Check sheet for the modelled part. Datum: model origin and axes. Units: mm. A direction names the side the tool comes from. Round coordinates to 2 decimals unless told otherwise and drop trailing zeros. Write each loop counter-clockwise with the first axis right and the second up, starting at its lowest first coordinate (ties: lowest second). Pieces come first, ordered by that corner, then holes. Notation, with made-up numbers: (70.5, -3) -> (110.5, -3) arc R21 ccw to (110.5, 20) -> close; hole circle Ø11 at (23, -8). An arc over 180 degrees is marked (long way). One line per item, written item: value.
from build123d import *

# Parameters (mm, degrees)
SKETCH_1_R             = 0.5
EXTRUDE_1_DEPTH        = 10
HOLE_WIZARD_M3_1_D     = 2.5
HOLE_WIZARD_M3_1_DEPTH = 18.5
HOLE_WIZARD_M3_1_TIP   = 0.751075774
SKETCH_4_R             = 0.5
EXTRUDE_2_DEPTH        = 10
HOLE_WIZARD_M3_2_D     = 2.5
HOLE_WIZARD_M3_2_DEPTH = 18.5
HOLE_WIZARD_M3_2_TIP   = 0.751075774
SKETCH_6_W             = 18
SKETCH_6_H             = 9
CUT_EXTRUDE_1_DEPTH    = 0.5
EXTRUDE_3_DEPTH        = 0.5
EXTRUDE_4_DEPTH        = 2
FILLET_4_R             = 1
SKETCH_10_R            = 1
EXTRUDE_5_DEPTH        = 1
SKETCH_11_W            = 12
SKETCH_11_H            = 7
EXTRUDE_6_DEPTH        = 0.1
SKETCH_12_R            = 1
EXTRUDE_7_DEPTH        = 1
SKETCH_13_R            = 1.75
EXTRUDE_8_DEPTH        = 7
DRAFT_1_ANGLE          = 5


with BuildPart() as part:
    # 草图1 → 凸台-拉伸1 (new body)
    with BuildSketch(Plane(origin=(0, 0, 0), x_dir=(1, 0, 0), z_dir=(0, 1, 0))):
        with BuildLine():
            Line((-12.5, 10), (-17.5, 5))
            Line((-17.5, 5), (-17.5, -7.5))
            ThreePointArc((-17.5, -7.5), (-16.767766953, -9.267766953), (-15, -10))
            Line((-15, -10), (15, -10))
            ThreePointArc((15, -10), (16.767766953, -9.267766953), (17.5, -7.5))
            Line((17.5, -7.5), (17.5, 9.5))
            ThreePointArc((17.5, 9.5), (17.353553391, 9.853553391), (17, 10))
            Line((17, 10), (-12.5, 10))
        make_face()
        with Locations((-15, -7.5)):
            Circle(SKETCH_1_R, mode=Mode.SUBTRACT)
    extrude(amount=EXTRUDE_1_DEPTH)

    # M3 螺纹孔1
    with Locations(Plane(origin=(10, 10, 7.5), x_dir=(0, 0, 1), z_dir=(0, 1, 0))):
        with Locations((0, 0)):
            Hole(HOLE_WIZARD_M3_1_D / 2, depth=HOLE_WIZARD_M3_1_DEPTH)
            with Locations((0, 0, -(HOLE_WIZARD_M3_1_DEPTH + HOLE_WIZARD_M3_1_TIP / 2))):  # 118° drill point
                Cone(0, HOLE_WIZARD_M3_1_D / 2, HOLE_WIZARD_M3_1_TIP, mode=Mode.SUBTRACT)

    # 草图4 → 凸台-拉伸2 (add)
    with BuildSketch(Plane.XZ):
        with Locations((-15, 7.5)):
            Circle(SKETCH_4_R)
    extrude(amount=-EXTRUDE_2_DEPTH)

    # M3 螺纹孔2
    with Locations(Plane(origin=(-15, 10, 7.5), x_dir=(0, 0, 1), z_dir=(0, 1, 0))):
        with Locations((0, 0)):
            Hole(HOLE_WIZARD_M3_2_D / 2, depth=HOLE_WIZARD_M3_2_DEPTH)
            with Locations((0, 0, -(HOLE_WIZARD_M3_2_DEPTH + HOLE_WIZARD_M3_2_TIP / 2))):  # 118° drill point
                Cone(0, HOLE_WIZARD_M3_2_D / 2, HOLE_WIZARD_M3_2_TIP, mode=Mode.SUBTRACT)

    # 草图6 → 切除-拉伸1 (cut)
    with BuildSketch(Plane.XY.offset(10)):
        with Locations((-2, 5)):
            Rectangle(SKETCH_6_W, SKETCH_6_H)
    extrude(amount=-CUT_EXTRUDE_1_DEPTH, mode=Mode.SUBTRACT)

    # 草图8 → 凸台-拉伸3 (add)
    with BuildSketch(Plane(origin=(17.5, 0, 0), x_dir=(0, 0, -1), z_dir=(1, 0, 0))):
        with BuildLine():
            Line((8, 8.5), (-6, 8.5))
            ThreePointArc((-6, 8.5), (-6.353553391, 8.353553391), (-6.5, 8))
            Line((-6.5, 8), (-6.5, 2))
            ThreePointArc((-6.5, 2), (-6.353553391, 1.646446609), (-6, 1.5))
            Line((-6, 1.5), (8, 1.5))
            ThreePointArc((8, 1.5), (8.353553391, 1.646446609), (8.5, 2))
            Line((8.5, 2), (8.5, 8))
            ThreePointArc((8.5, 8), (8.353553391, 8.353553391), (8, 8.5))
        make_face()
    extrude(amount=EXTRUDE_3_DEPTH)

    # 草图9 → 凸台-拉伸4 (add)
    with BuildSketch(Plane(origin=(18, 0, 0), x_dir=(0, 0, -1), z_dir=(1, 0, 0))):
        with BuildLine():
            Line((-2, 6.5), (-2, 3.5))
            ThreePointArc((-2, 3.5), (-3.5, 2), (-5, 3.5))
            Line((-5, 3.5), (-5, 6.5))
            ThreePointArc((-5, 6.5), (-3.5, 8), (-2, 6.5))
        make_face()
    extrude(amount=EXTRUDE_4_DEPTH)

    # 圆角4
    fillet_4_edges = [part.edges().sort_by_distance(p)[0] for p in [
        (20, 8, 3.5),
        (20, 5, 5),
        (20, 2, 3.5),
        (20, 5, 2),
    ]]
    fillet(fillet_4_edges, radius=FILLET_4_R)

    # 草图10 → 凸台-拉伸5 (add)
    with BuildSketch(Plane(origin=(18, 0, 0), x_dir=(0, 0, -1), z_dir=(1, 0, 0))):
        with Locations((3.5, 5)):
            Circle(SKETCH_10_R)
    extrude(amount=EXTRUDE_5_DEPTH)

    # 草图11 → 凸台-拉伸6 (add)
    with BuildSketch(Plane(origin=(0, 0, -10), x_dir=(-1, 0, 0), z_dir=(0, 0, -1))):
        with Locations((-2.25, 5)):
            Rectangle(SKETCH_11_W, SKETCH_11_H)
    extrude(amount=EXTRUDE_6_DEPTH)

    # 草图12 → 凸台-拉伸7 (add)
    with BuildSketch(Plane(origin=(0, 0, -10), x_dir=(-1, 0, 0), z_dir=(0, 0, -1))):
        with Locations((-11.25, 5)):
            Circle(SKETCH_12_R)
        with Locations((6.75, 5)):
            Circle(SKETCH_12_R)
    extrude(amount=EXTRUDE_7_DEPTH)

    # 草图13 → 凸台-拉伸8 (add)
    with BuildSketch(Plane(origin=(-11.25, 0, -11.25), x_dir=(-0.707106781, 0, 0.707106781), z_dir=(-0.707106781, 0, -0.707106781))):
        with Locations((5.303300859, 5)):
            Circle(SKETCH_13_R)
    extrude(amount=EXTRUDE_8_DEPTH)

    # 拔模1
    draft_1_faces = [part.faces().sort_by_distance(p)[0] for p in [
        (-16.237436867, 5, -11.212310601),
    ]]
    draft(draft_1_faces, Plane(origin=(-19.949747468, 5, -12.449747468), x_dir=(-0.707106781, 0, 0.707106781), z_dir=(-0.707106781, 0, -0.707106781)), DRAFT_1_ANGLE)


solid = part.part
Item 1: Sectioned sample at C-C (x = -6.75). Enter the section's corners in (y, z), then the cut area to 4 significant figures.
Result set:
outline: (0, -10) -> (4, -10) -> (4, -11) -> (6, -11) -> (6, -10) -> (10, -10) -> (10, 10) -> (9.5, 10) -> (9.5, 9.5) -> (0.5, 9.5) -> (0.5, 10) -> (0, 10) -> close
area: 197.5 mm^2
Item 2: Depth check by flat-ended pin: pin 1 (1 mm diameter, centred on y = 4.5, z = -4, fed in from +X); pin 2 (2 mm diameter, centred on y = 5, z = 3, fed in from -X); pin 3 (4.5 mm diameter, centred on x = -1.5, y = 4.5, fed in from +Z). Enter the tip coordinate at first touch or a pass-through.
Result set:
pin 1: x = 19
pin 2: x = -17.5
pin 3: z = 9.5
Item 3: Release check for a two-part mould opening along X. For faces 4 (the flat face through (-17.5, 5, 1)), 5 (the flat face through (0, 0, 0)), 6 (the conical face through (-16.366, 6.393, -11.014)) record: pulls with the +X half, pulls with the -X half, needs draft (parallel to the pull), parting line crosses it, or undercut.
Result set:
face 4: pulls with the -X half
face 5: needs draft
face 6: undercut
Item 4: Tool access check on faces 1 (the cylindrical face through (18.5, 8, 3.5)), 2 (the cylindrical face through (18.493, 5.676, -2.763)), 3 (the cylindrical face through (-6.013, 5.676, -10.493)). Record the directions out of +Z, -Z, +X, -X, +Y, -Y that give a thin tool (end or side, any length) a straight path to the whole face; none if there is none.
Result set:
face 1: +X, +Y
face 2: +X
face 3: -Z
Item 5: Sectioned sample at D-D (y = 5.5). State how many separate pieces and enclosed holes the cut face has, then the cut area to 3 significant figures.
Result set:
separate pieces: 1
enclosed holes: 2
area: 713 mm^2
Item 6: Material ranges on line 1 along X through (y, z) = (5.75, 7.5); line 2 along X through (y, z) = (5, -3.5); line 3 along X through (y, z) = (4.25, -9.25), recorded low to high.
Result set:
line 1: -17.5 to -16.25, -13.75 to 8.75, 11.25 to 17.5
line 2: -17.5 to 19
line 3: -19.35 to -13.62, -13.25 to 17.5
Item 7: Sectioned sample at B-B (z = 5.5). Enter the section's corners in (x, y), then the cut area to 4 significant figures.
Result set:
outline: (-17.5, 0) -> (17.5, 0) -> (17.5, 1.5) -> (18, 1.5) -> (18, 8.5) -> (17.5, 8.5) -> (17.5, 10) -> (-17.5, 10) -> close
area: 353.5 mm^2
Item 8: Sectioned sample at A-A (x = -2.5). Enter the section's corners in (y, z), then the cut area to 3 significant figures.
Result set:
outline: (0, -10) -> (1.5, -10) -> (1.5, -10.1) -> (8.5, -10.1) -> (8.5, -10) -> (10, -10) -> (10, 10) -> (9.5, 10) -> (9.5, 9.5) -> (0.5, 9.5) -> (0.5, 10) -> (0, 10) -> close
area: 196 mm^2
